Input: part model. Units: mm. Frame: model coordinates. Face numbers are marked on the shaded views. A direction names the side the tool comes from. Coordinates: 2 decimals unless noted, no trailing zeros. Write each loop counter-clockwise with the first axis right and the second up, starting at its lowest first coordinate (ties: lowest second). Pieces come first, ordered by that corner, then holes.
from build123d import *

# Parameters (mm, degrees)
PAD_DEPTH       = 30
SKETCH001_W     = 30
SKETCH001_H     = 25
SKETCH001_W_2   = 8
SKETCH001_H_2   = 10
POCKET_DEPTH    = 67.001
SKETCH002_W     = 24
SKETCH002_H     = 5
PAD001_DEPTH    = 25
SKETCH003_R     = 2
POCKET001_DEPTH = 5
PAD002_DEPTH    = 4


with BuildPart() as part:
    # Sketch → Pad (new body)
    with BuildSketch(Plane.XY):
        Polygon((-28.5, 0), (-28.5, 40), (28.5, 40), (28.5, 0), (33.5, 0), (33.5, 45), (12, 75), (-12, 75), (-33.5, 45), (-33.5, 0), align=None)
    extrude(amount=PAD_DEPTH)

    # Sketch001 (on Face7 of Pad) → Pocket (cut, through all)
    with BuildSketch(Plane.YZ.offset(33.5)):
        with Locations((60, 12.5)):
            Rectangle(SKETCH001_W, SKETCH001_H)
        with Locations((4, 15)):
            Rectangle(SKETCH001_W_2, SKETCH001_H_2)
    extrude(amount=-POCKET_DEPTH, mode=Mode.SUBTRACT)

    # Sketch002 (on Face19 of Pocket) → Pad001 (join)
    with BuildSketch(Plane(origin=(0, 0, 25), x_dir=(1, 0, 0), z_dir=(0, 0, -1))):
        with Locations((0, -72.5)):
            Rectangle(SKETCH002_W, SKETCH002_H)
    extrude(amount=PAD001_DEPTH)

    # Sketch003 (on Face23 of Pad001) → Pocket001 (cut)
    with BuildSketch(Plane(origin=(0, 75, 0), x_dir=(-1, 0, 0), z_dir=(0, 1, 0))):
        with Locations((0, 10)):
            Circle(SKETCH003_R)
    extrude(amount=-POCKET001_DEPTH, mode=Mode.SUBTRACT)

    # Sketch004 (on Face12 of Pocket001) → Pad002 (join)
    with BuildSketch(Plane.XZ):
        Polygon((32.5, 20), (33.5, 24), (36.5, 20), (36.5, 10), (33.5, 6), (32.5, 10), align=None)
        Polygon((-32.5, 20), (-33.5, 24), (-36.5, 20), (-36.5, 10), (-33.5, 6), (-32.5, 10), align=None)
    extrude(amount=-PAD002_DEPTH)


solid = part.part
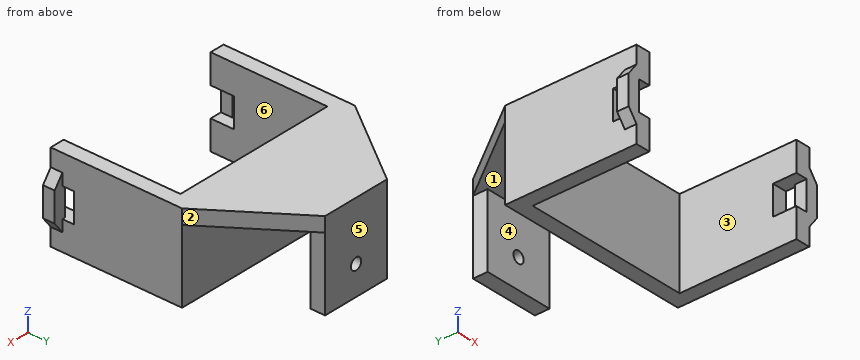
Item 1: Pull-direction query (X, two-part tool) for the marked faces 1, 2 and 3; classes: released by +X, released by -X, zero draft, split by the parting line, or undercut.
Item 2: Section query B-B, the plane x = 0. Return loops of the section in (y, z).
Item 3: Section query A-A, the plane z = 17.5. Return loops of the section in (x, y).
Item 4: Section query C-C, the plane y = 6.5. Return loops of the section in (x, z), then the cut area to 3 significant figures.
Item 5: Material intervals for line 1 (Z direction, x = -30, y = 5); line 2 (X direction, y = 11.5, z = 20.75); line 3 (Y direction, x = 0, z = 22.25), sorted ascending.
Item 6: Section query D-D, the plane y = 15. Return loops of the section in (x, z).
Item 7: Access query for the marked faces 4, 5 and 6. Directions: +Z, -Z, +X, -X, +Y, -Y. A direction counts if a zero-diameter tool reaches every point of the face in a straight line with its end or side. Return the directions, or none.
Item 8: Pin query (flat end, axial travel): pin 1 Ø2.5 at (y, z) = (73.5, 17) entering from +X; pin 2 Ø5.5 at (x, z) = (30.5, 16.5) entering from -Y; pin 3 Ø2.5 at (y, z) = (73.5, 13) entering from -X; pin 4 Ø1.2 at (x, z) = (-35, 12) entering from +Y. Return the tip coordinate at first contact, or that it passes through.
The answers:
1. face 1: zero draft
1. face 2: released by +X
1. face 3: undercut
2. outline: (40, 0) - (45, 0) - (45, 25) - (70, 25) - (70, 12) - (75, 12) - (75, 30) - (40, 30) - close; (70, 0) - (75, 0) - (75, 8) - (70, 8) - close
3. outline: (-36.5, 0) - (-32.5, 0) - (-32.5, 4) - (-36.5, 4) - close; (-33.5, 8) - (-28.5, 8) - (-28.5, 40) - (28.5, 40) - (28.5, 8) - (33.5, 8) - (33.5, 45) - (-33.5, 45) - close; (-12, 70) - (12, 70) - (12, 75) - (-12, 75) - close; (32.5, 0) - (36.5, 0) - (36.5, 4) - (32.5, 4) - close
4. outline: (-33.5, 0) - (-28.5, 0) - (-28.5, 10) - (-33.5, 10) - close; (-33.5, 20) - (-28.5, 20) - (-28.5, 30) - (-33.5, 30) - close; (28.5, 0) - (33.5, 0) - (33.5, 10) - (28.5, 10) - close; (28.5, 20) - (33.5, 20) - (33.5, 30) - (28.5, 30) - close
4. area: 200 mm2
5. line 1: z = 0 to 10, 20 to 30
5. line 2: x = -33.5 to -28.5, 28.5 to 33.5
5. line 3: y = 40 to 45, 70 to 75
6. outline: (-33.5, 0) - (-28.5, 0) - (-28.5, 30) - (-33.5, 30) - close; (28.5, 0) - (33.5, 0) - (33.5, 30) - (28.5, 30) - close
7. face 4: -Z, +X, -X
7. face 5: +Z, -Z, +X, -X, +Y
7. face 6: +Z, -Z, -Y
8. pin 1: stops at x = 12
8. pin 2: stops at y = 0
8. pin 3: stops at x = -12
8. pin 4: stops at y = 4
